Can you work these out from the model? Positions are in its coordinate system, mm. Face numbers are marked on the shaded views. A direction names the side the tool comes from. Give positions to 0.01 mm unless a question says otherwise; leave off trailing zeros. Loops run counter-clockwise (first coordinate to the right, second up) from the corner with the lowest first, then second, coordinate; pieces in that order, holes last. Notation, with made-up numbers: (81, 6) - (119, 6) arc R28 ccw to (119, 28) - close; hole circle Ø10 at (17, 56). An arc over 180 degrees is marked (long way). Answer as a JSON object with one key per item and string values. Group by question number.
Item 1: Suppose I cut it at C-C on y = 8.5. Write out the boundary of the cut face in (x, z), and give its area (3 significant figures).
Item 2: Please list where these lines run through material, in increasing order: L1, parallel to Z at x = 11.5, y = 13.15; L2, parallel to Z at x = -5.75, y = 12.75; L3, parallel to X at y = 13.25, z = 0.
Item 3: Will these pins go through, and if not, where does the flat tip stop? pin 1 (6.5 mm diameter, centred on x = 11.5, z = 0, fed in from -Y); pin 2 (9 mm diameter, centred on x = -5.75, z = -9.96, fed in from -Y); pin 3 (2 mm diameter, centred on x = 12, z = 1, fed in from -Y); pin 4 (3 mm diameter, centred on y = 10.5, z = 4.5, fed in from +X).
Item 4: Which directions (+Z, -Z, +X, -X, +Y, -Y) give clear straight access to the entire face, cutting with the end or side of a thin tool? Please do the marked faces 4, 5 and 6.
Item 5: Thinking about a two-plate mould opening in X: for the marked faces 1, 2 and 3, which applies, pulls with the +X half, pulls with the -X half, needs draft (parallel to the pull), parting line crosses it, or undercut?
Item 6: Suppose I cut it at A-A on x = 11.5. Write out the boundary of the cut face in (y, z).
Item 7: Suppose I cut it at D-D on x = -5.75. Write out the boundary of the cut face in (y, z).
Item 8: Suppose I cut it at B-B on z = 0. Write out the boundary of the cut face in (x, y).
Autodesk Inventor part; units mm, degrees
ref_plane "YZ Plane" through (0, 0, 0) normal (1, 0, 0) x (0, 1, 0)
ref_plane "XZ Plane" through (0, 0, 0) normal (0, 1, 0) x (-1, 0, 0)
ref_plane "XY Plane" through (0, 0, 0) normal (0, 0, 1) x (1, 0, 0)
sketch "Sketch1" plane through (0, 0, 0) normal (0, 1, 0) x (-1, 0, 0)
  circle A0 centre (0, 0) radius 11.5 construction
  line L0 (0, 0) -> (5.75, 9.9593) construction
  line L1 (0, 0) -> (5.75, -9.9593) construction
  line L2 (11.5, 0) -> (0, 0) construction
  circle A1 centre (5.75, 9.9593) radius 1.75
  circle A2 centre (5.75, -9.9593) radius 1.75
  circle A3 centre (0, 0) radius 22.5
  line L3 (14.1421, 17.5) -> (-14.1421, 17.5)
  line L4 (14.1421, -17.5) -> (-14.1421, -17.5)
  line L5 (-22.5, -22.5) -> (22.5, -22.5)
  line L6 (22.5, -22.5) -> (22.5, 22.5)
  line L7 (22.5, 22.5) -> (-22.5, 22.5)
  line L8 (-22.5, 22.5) -> (-22.5, -22.5)
  line L9 (-22.5, -22.5) -> (22.5, 22.5) construction
  line L10 (22.5, -22.5) -> (-22.5, 22.5) construction
  circle A4 centre (-11.5, 0) radius 2.75
  circle A5 centre (5.75, 9.9593) radius 2.75
  circle A6 centre (5.75, -9.9593) radius 2.75
  point P0 (-22.5, 0)
  point P1 (22.5, 0)
  dimension "d0" = 23
  dimension "d1" = 60
  dimension "d2" = 3.5
  dimension "d6" = 35
  dimension "d7" = 45
  dimension "d16" = 5.5
sketch "Sketch2" plane through (0, 0, 0) normal (1, 0, 0) x (0, 1, 0)
  line L0 (0, 17.5) -> (0, 6.5)
  line L1 (0, 6.5) -> (10, 6.5)
  line L2 (10, 6.5) -> (10, -6.5)
  line L3 (10, -6.5) -> (0, -6.5)
  line L4 (0, -6.5) -> (0, -17.5)
  line L5 (11, -17.5) -> (15, -17.5)
  line L6 (15, -17.5) -> (15, 17.5)
  line L7 (15, 17.5) -> (0, 17.5)
  line L8 (11, -17.5) -> (0, -17.5)
  line L9 (0, 0) -> (15, 0) construction
  point P0 (0, -17.5)
  dimension "d5" = 15
  dimension "d14" = 13
  dimension "d15" = 5
extrude "Extrusion1" add sketch "Sketch2" along normal mid plane 45
extrude "Extrusion2" cut sketch "Sketch1" along normal through all contours L6 L5 A3 | A3 L7 L6 | L3 A3 | A3 L4 | A3 L8 L7 | L5 L8 A3
extrude "Extrusion3" cut sketch "Sketch1" along normal through all contours A1 | A2
extrude "Extrusion4" cut sketch "Sketch1" along normal through all contours A4
extrude "Extrusion5" cut sketch "Sketch1" against normal blind 8 from surface at 15 contours A1 | A2 | A5 | A6
properties part number "back_hip_cable_protector"
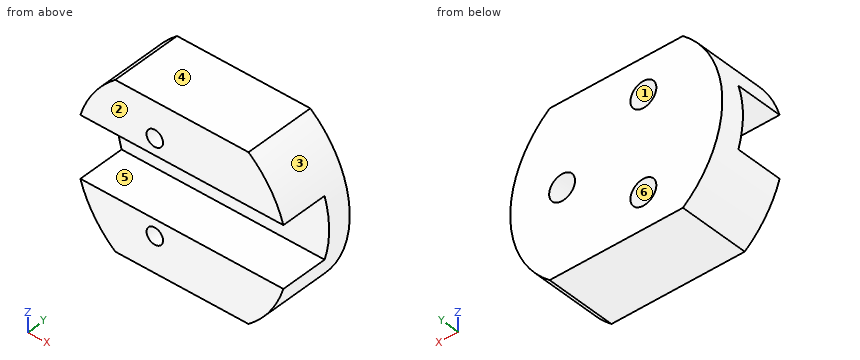
Worked out:
{
 "1": {"outline": "(-21.54, -6.5) arc R22.5 ccw to (-14.14, -17.5) - (14.14, -17.5) arc R22.5 ccw to (21.54, -6.5) - close; (-21.54, 6.5) - (21.54, 6.5) arc R22.5 ccw to (14.14, 17.5) - (-14.14, 17.5) arc R22.5 ccw to start; hole circle Ø5.5 at (-5.75, -9.96); hole circle Ø5.5 at (-5.75, 9.96)", "area": "773 mm2"},
 "2": {"L1": "z = -17.5 to -2.75, 2.75 to 17.5", "L2": "z = -17.5 to -12.71, -7.21 to 7.21, 12.71 to 17.5", "L3": "x = -22.5 to 8.75, 14.25 to 22.5"},
 "3": {"pin 1": "stops at y = 10", "pin 2": "stops at y = 0", "pin 3": "passes through", "pin 4": "stops at x = 22.3"},
 "4": {"face 4": "+Z, +X, -X, +Y, -Y", "face 5": "+X, -X, -Y", "face 6": "+Y"},
 "5": {"face 1": "undercut", "face 2": "needs draft", "face 3": "pulls with the +X half"},
 "6": {"outline": "(0, -17.5) - (15, -17.5) - (15, -2.75) - (10, -2.75) - (10, -6.5) - (0, -6.5) - close; (0, 6.5) - (10, 6.5) - (10, 2.75) - (15, 2.75) - (15, 17.5) - (0, 17.5) - close"},
 "7": {"outline": "(0, -17.5) - (15, -17.5) - (15, -12.71) - (7, -12.71) - (7, -11.71) - (0, -11.71) - close; (0, -8.21) - (7, -8.21) - (7, -7.21) - (15, -7.21) - (15, 7.21) - (7, 7.21) - (7, 8.21) - (0, 8.21) - (0, 6.5) - (10, 6.5) - (10, -6.5) - (0, -6.5) - close; (0, 11.71) - (7, 11.71) - (7, 12.71) - (15, 12.71) - (15, 17.5) - (0, 17.5) - close"},
 "8": {"outline": "(-22.5, 10) - (8.75, 10) - (8.75, 15) - (-22.5, 15) - close; (14.25, 10) - (22.5, 10) - (22.5, 15) - (14.25, 15) - close"}
}
